from build123d import *


with BuildPart() as part:
    # Sketch1 → Revolve1 (revolve)
    with BuildSketch(Plane.XY, mode=Mode.PRIVATE) as revolve1_sk:
        with BuildLine():
            Line((5.5, 0), (5.5, 2.5))
            Line((5.5, 2.5), (3, 2.5))
            Line((3, 2.5), (2.5, 3.87373871))
            Line((2.5, 3.87373871), (2.5, 92.5))
            Line((2.5, 92.5), (1.5, 92.5))
            Line((1.5, 92.5), (1.5, 94.5))
            Line((1.5, 94.5), (2, 94.5))
            Line((2, 94.5), (2, 100.5))
            Line((2, 100.5), (0, 100.5))
            Line((0, 100.5), (0, -5.5))
            ThreePointArc((0, -5.5), (3.889087297, -3.889087297), (5.5, 0))
        make_face()
    revolve(revolve1_sk.sketch.rotate(Axis((0, 0, 0), (0, 1, 0)), 90), axis=Axis((0, 0, 0), (0, 1, 0)))


solid = part.part
Here's how the part is built. I have some questions about the finished solid (model axes, mm). A direction names the side the tool comes from. Coordinates: 2 decimals unless noted, no trailing zeros. Write each loop counter-clockwise with the first axis right and the second up, starting at its lowest first coordinate (ties: lowest second). Pieces come first, ordered by that corner, then holes.
Item 1: If we mould it in two halves opening along Y, with no side actions, what happens to faces 1 (the cylindrical face through (-0.45, 93.51, -1.43)), 2 (the flat face through (0, 100.5, 0)), 3 (the flat face through (0, 92.5, -2)), 4 (the cylindrical face through (-0.1, 48.8, 2.5))? For each: +Y half, -Y half, draft (parallel to the pull), parting line (faces both ways), or undercut.
Item 2: If I drill on line 1 (X direction, y = 38, z = 2); line 2 (Y direction, x = -1.75, z = 0.25), over which ranges is the centre line in solid material (lowest first)?
Item 3: Will these pins go through, and if not, where does the flat tip stop? pin 1 (1.5 mm diameter, centred on y = 40, z = 0.5, fed in from +X); pin 2 (4 mm diameter, centred on x = 1.5, y = 76.5, fed in from +Z); pin 3 (1.5 mm diameter, centred on y = 21.5, z = -3, fed in from +X).
Item 4: On a 3-axis mill with a long thin cutter (end or side, diameter ignored), from which of +Z, -Z, +X, -X, +Y, -Y can I reach the whole of each face in a straight line? I mean faces 5 (the flat face through (2.4, 2.5, -2.4)), 6 (the cylindrical face through (5.37, 1.27, 1.19)). Say none if no direction works.
Item 5: I want a section at C-C on y = 70.5. Write out the boundary of the cut face in (x, z), and give its area (3 significant figures).
Item 6: I want a section at B-B on x = 0. Write out the boundary of the cut face in (y, z), and give its area (3 significant figures).
Item 7: I want a section at D-D on z = 4.5. Write out the boundary of the cut face in (x, y), and give its area (3 significant figures).
Item 8: I want a section at A-A on z = 0. Write out the boundary of the cut face in (x, y), and give its area (3 significant figures).
Findings below:
1. face 1: undercut
1. face 2: +Y half
1. face 3: undercut
1. face 4: draft
2. line 1: x = -1.5 to 1.5
2. line 2: y = -5.21 to 92.5, 94.5 to 100.5
3. pin 1: stops at x = 2.5
3. pin 2: stops at z = 2.5
3. pin 3: stops at x = 1.09
4. face 5: +Y
4. face 6: +Y, -Y
5. outline: circle Ø5 at (0, 0)
5. area: 19.6 mm2
6. outline: (0, -5.5) - (2.5, -5.5) - (2.5, -3) - (3.87, -2.5) - (92.5, -2.5) - (92.5, -1.5) - (94.5, -1.5) - (94.5, -2) - (100.5, -2) - (100.5, 2) - (94.5, 2) - (94.5, 1.5) - (92.5, 1.5) - (92.5, 2.5) - (3.87, 2.5) - (2.5, 3) - (2.5, 5.5) - (0, 5.5) arc R5.5 ccw to start
6. area: 556 mm2
7. outline: (-3.16, 0) arc R3.16 ccw to (3.16, 0) - (3.16, 2.5) - (-3.16, 2.5) - close
7. area: 31.5 mm2
8. outline: (-5.5, 0) arc R5.5 ccw to (5.5, 0) - (5.5, 2.5) - (3, 2.5) - (2.5, 3.87) - (2.5, 92.5) - (1.5, 92.5) - (1.5, 94.5) - (2, 94.5) - (2, 100.5) - (-2, 100.5) - (-2, 94.5) - (-1.5, 94.5) - (-1.5, 92.5) - (-2.5, 92.5) - (-2.5, 3.87) - (-3, 2.5) - (-5.5, 2.5) - close
8. area: 556 mm2
